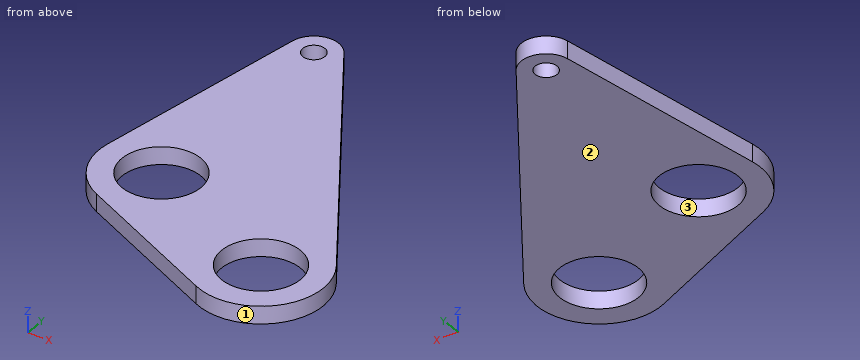
Autodesk Inventor part; units mm, degrees
ref_plane "YZ Plane" through (0, 0, 0) normal (1, 0, 0) x (0, 1, 0)
ref_plane "XZ Plane" through (0, 0, 0) normal (0, 1, 0) x (-1, 0, 0)
ref_plane "XY Plane" through (0, 0, 0) normal (0, 0, 1) x (1, 0, 0)
sketch "Sketch1" plane through (0, 0, 0) normal (0, 0, 1) x (1, 0, 0)
  circle A0 centre (0, 0) radius 14.2875
  circle A1 centre (53.1212, -24.3113) radius 14.2875
  circle A2 centre (0, 80) radius 4
  line L0 (0, 80) -> (0, 0) construction
  line L1 (0, 0) -> (53.1212, -24.3113) construction
  circle A3 centre (53.1212, -24.3113) radius 15.5575
  circle A4 centre (0, 0) radius 15.5575
  arc A5 (43.7339, -44.8228) -> (71.9014, -11.8155) centre (53.1212, -24.3113) ccw
  arc A6 (-22.2312, 3.8228) -> (-9.3872, -20.5115) centre (0, 0) ccw
  arc A7 (7.4929, 84.9856) -> (-8.8698, 81.5252) centre (0, 80) ccw
  line L2 (-8.8698, 81.5252) -> (-22.2312, 3.8228)
  line L3 (-9.3872, -20.5115) -> (43.7339, -44.8228)
  line L4 (71.9014, -11.8155) -> (7.4929, 84.9856)
  dimension "d0" = 8
  dimension "d1" = 28.575
  dimension "d4" = 28.575
  dimension "d5" = 58.42
  dimension "d6" = 114.592
  dimension "d7" = 80
  dimension "d8" = 31.115
  dimension "d9" = 31.115
  dimension "d10" = 5
  dimension "d11" = 7
  dimension "d13" = 7
extrude "Extrusion1" add sketch "Sketch1" along normal blind 6.35 contours A3 | A4 | L3 A6 L2 A7 L4 A5
equation "\"d4\" = d1"
equation "\"d6\" = d2"
equation "\"d9\" = d8"
equation "\"d13\" = d11"
properties part number "sussy pivot"
Build history of the part. All positions in model axes, mm. Face numbers are marked on the shaded views. Round coordinates to 2 decimals unless told otherwise and drop trailing zeros. Write each loop counter-clockwise with the first axis right and the second up, starting at its lowest first coordinate (ties: lowest second). Pieces come first, ordered by that corner, then holes. Notation, with made-up numbers: (9, 46) -> (56, 46) arc R31 cw to (56, 75) -> close; hole circle Ø2 at (-1, 49). An arc over 180 degrees is marked (long way). Use one line per item in the form item = value.
Q1. Band-saw the part on B-B, the plane x = 54.5. Write the cut outline in (y, z), then the cut area to 3 significant figures.
Conclusion:
outline = (-46.83, 0) -> (-38.53, 0) -> (-38.53, 6.35) -> (-46.83, 6.35) -> close; (-10.09, 0) -> (14.34, 0) -> (14.34, 6.35) -> (-10.09, 6.35) -> close
area = 208 mm²
Q2. Band-saw the part on D-D, the plane z = 2.25. Write the cut outline in (x, y) (1 decimal), then the cut area to 3 significant figures.
Conclusion:
outline = (-22.2, 3.8) arc R22.6 ccw to (-9.4, -20.5) -> (43.7, -44.8) arc R22.6 ccw to (71.9, -11.8) -> (7.5, 85) arc R9 ccw to (-8.9, 81.5) -> close; hole circle Ø28.6 at (0, 0); hole circle Ø8 at (0, 80); hole circle Ø28.6 at (53.1, -24.3)
area = 6,280 mm²
Q3. Band-saw the part on A-A, the plane y = 7. Write the cut outline in (x, z), then the cut area to 3 significant figures.
Conclusion:
outline = (-21.68, 0) -> (-12.46, 0) -> (-12.46, 6.35) -> (-21.68, 6.35) -> close; (12.46, 0) -> (59.38, 0) -> (59.38, 6.35) -> (12.46, 6.35) -> close
area = 357 mm²
Q4. Band-saw the part on C-C, the plane x = 0. Write the cut outline in (y, z), then the cut area to 3 significant figures.
Conclusion:
outline = (-24.81, 0) -> (-14.29, 0) -> (-14.29, 6.35) -> (-24.81, 6.35) -> close; (14.29, 0) -> (76, 0) -> (76, 6.35) -> (14.29, 6.35) -> close; (84, 0) -> (89, 0) -> (89, 6.35) -> (84, 6.35) -> close
area = 490 mm²
Q5. Two-plate mould, pull along X, no slides. Class the marked faces 1, 2 and 3: released by +X, released by -X, zero draft, split by the parting line, or undercut.
Conclusion:
face_1 = split by the parting line
face_2 = zero draft
face_3 = undercut
Q6. Drop flat-ended pins along their axis: P1, Ø1.5, axis at x = -6.5, z = 1.5, coming from the -Y side; P2, Ø2, axis at x = 38.5, z = 5.5, coming from the -Y side. Give the stop position or say it passes through.
Conclusion:
P1 = -22.18
P2 = -42.89
Q7. Drill centre lines: L1, parallel to Y at x = -0.5, z = 3.25; L2, parallel to Y at x = 0, z = 1.75; L3, parallel to X at y = -36.5, z = 5.25. Where is each one in solid material? Low to high.
Conclusion:
L1 = -24.58 to -14.28, 14.28 to 76.03, 83.97 to 88.99
L2 = -24.81 to -14.29, 14.29 to 76, 84 to 89
L3 = 25.55 to 45.67, 60.58 to 72.1
